from build123d import *

# Parameters (mm, degrees)
SKETCH1_R           = 80
SKETCH1_R_2         = 2.6
BOSS_EXTRUDE1_DEPTH = 1.5
SKETCH2_R           = 2.6
CUT_EXTRUDE1_DEPTH  = 10
CIRPATTERN1_COUNT   = 4


with BuildPart() as part:
    # Sketch1 → Boss-Extrude1 (new body)
    with BuildSketch(Plane.XY):
        Circle(SKETCH1_R)
        with Locations((-46.280707897, 55.155199905)):
            Circle(SKETCH1_R_2, mode=Mode.SUBTRACT)
        with Locations((-46.280707897, -55.155199905)):
            Circle(SKETCH1_R_2, mode=Mode.SUBTRACT)
        with Locations((46.280707897, -55.155199905)):
            Circle(SKETCH1_R_2, mode=Mode.SUBTRACT)
        with Locations((46.280707897, 55.155199905)):
            Circle(SKETCH1_R_2, mode=Mode.SUBTRACT)
        with Locations((0, 40)):
            Circle(SKETCH1_R_2, mode=Mode.SUBTRACT)
        with Locations((40, 0)):
            Circle(SKETCH1_R_2, mode=Mode.SUBTRACT)
        with Locations((0, -40)):
            Circle(SKETCH1_R_2, mode=Mode.SUBTRACT)
        with Locations((-40, 0)):
            Circle(SKETCH1_R_2, mode=Mode.SUBTRACT)
    extrude(amount=BOSS_EXTRUDE1_DEPTH)

    # Sketch2 → Cut-Extrude1 (cut)
    with BuildSketch(Plane(origin=(0, 0, 0), x_dir=(-1, 0, 0), z_dir=(0, 0, -1))):
        with Locations((-11.570176974, 13.788799976)):
            Circle(SKETCH2_R)
    cut_extrude1 = extrude(amount=-CUT_EXTRUDE1_DEPTH, mode=Mode.SUBTRACT)

    # CirPattern1: Cut-Extrude1 ×4 about axis
    cirpattern1_axis = Axis((0, 0, 0), (0, 0, 1))
    for i in range(1, CIRPATTERN1_COUNT):
        add(cut_extrude1.rotate(cirpattern1_axis, i * 360 / CIRPATTERN1_COUNT), mode=Mode.SUBTRACT)


solid = part.part
Geometry check sheet. Reference: the model listing, model coordinates, mm. Give positions to 0.01 mm unless a question says otherwise; leave off trailing zeros. Order: outer loops, then holes, each group sorted by start corner. A loop starts at its lowest first (then second) coordinate and runs counter-clockwise, first axis right, second up. Notation, with made-up numbers: M 28,43 L 76,43 A20 ccw 76,60 Z; hole C -6.75,-20 d6. An arc over 180 degrees is marked long. Use a Markdown table: item, result.
Item 1: Draft check along Y on faces 1 (the cylindrical face through (-17.34, -78.1, 0.74)), 2 (the flat face through (-1, 1, 1.5)), 3 (the cylindrical face through (-11.25, 12.13, 0.74)). Enter one of: +Y half, -Y half, draft (parallel to the pull), parting line (faces both ways), or undercut.
Answers follow:
| item | result |
|---|---|
| face 1 | parting line |
| face 2 | draft |
| face 3 | undercut |
Item 2: Section check A-A (x = 0). Record the cut outline in (y, z).
Answers follow:
| item | result |
|---|---|
| outline | M -80,0 L -42.6,0 L -42.6,1.5 L -80,1.5 Z; M -37.4,0 L 37.4,0 L 37.4,1.5 L -37.4,1.5 Z; M 42.6,0 L 80,0 L 80,1.5 L 42.6,1.5 Z |
Item 3: Material ranges on line 1 along Y through (x, z) = (0, 0.35); line 2 along Y through (x, z) = (-40, 0.75); line 3 along X through (y, z) = (-41.5, 1.1), recorded low to high.
Answers follow:
| item | result |
|---|---|
| line 1 | y = -80 to -42.6, -37.4 to 37.4, 42.6 to 80 |
| line 2 | y = -69.28 to -2.6, 2.6 to 69.28 |
| line 3 | x = -68.39 to -2.12, 2.12 to 68.39 |
Item 4: Section check D-D (z = 0.5). State how many separate pieces and enclosed holes the cut face has, and give its area (3 significant figures).
Answers follow:
| item | result |
|---|---|
| separate pieces | 1 |
| enclosed holes | 12 |
| area | 19,900 mm2 |
Item 5: Section check C-C (y = 40). Record the cut outline in (x, z), and give its area (3 significant figures).
Answers follow:
| item | result |
|---|---|
| outline | M -69.28,0 L -2.6,0 L -2.6,1.5 L -69.28,1.5 Z; M 2.6,0 L 69.28,0 L 69.28,1.5 L 2.6,1.5 Z |
| area | 200 mm2 |
